from build123d import *

# Parameters (mm, degrees)
SKETCH1_W           = 32
SKETCH1_H           = 20
SKETCH1_R           = 1.6
BOSS_EXTRUDE1_DEPTH = 2
SKETCH3_W           = 40
SKETCH3_H           = 9
SKETCH3_R           = 1.45
BOSS_EXTRUDE2_DEPTH = 4
CUT_EXTRUDE1_DEPTH  = 2
FILLET1_R           = 10
CHAMFER1_SIZE       = 1
CUT_EXTRUDE2_REACH  = 28.019
SKETCH12_R          = 1.45
SKETCH12_R_2        = 0.95
FILLET2_R           = 1


with BuildPart() as part:
    # Sketch1 → Boss-Extrude1 (new body)
    with BuildSketch(Plane(origin=(0, 0, 0), x_dir=(1, 0, 0), z_dir=(0, 1, 0))):
        Rectangle(SKETCH1_W, SKETCH1_H)
        with Locations(Location((-5, 7.5, 0), (0, 0, 270))):
            Circle(SKETCH1_R, mode=Mode.SUBTRACT)
        with Locations(Location((5, 7.5, 0), (0, 0, 270))):
            Circle(SKETCH1_R, mode=Mode.SUBTRACT)
        with Locations(Location((-5, -7.5, 0), (0, 0, 270))):
            Circle(SKETCH1_R, mode=Mode.SUBTRACT)
        with Locations(Location((5, -7.5, 0), (0, 0, 270))):
            Circle(SKETCH1_R, mode=Mode.SUBTRACT)
    extrude(amount=BOSS_EXTRUDE1_DEPTH)

    # Sketch3 → Boss-Extrude2 (add)
    with BuildSketch(Plane.XY.offset(10)):
        with Locations((0, -2.5)):
            Rectangle(SKETCH3_W, SKETCH3_H)
        with Locations((0, -2.5)):
            Circle(SKETCH3_R, mode=Mode.SUBTRACT)
    extrude(amount=BOSS_EXTRUDE2_DEPTH)

    # Sketch4 → Cut-Extrude1 (cut)
    with BuildSketch(Plane(origin=(0, 0, 10), x_dir=(-1, 0, 0), z_dir=(0, 0, -1))):
        with BuildLine():
            Line((-16, 2), (-20, 2))
            Line((-20, 2), (-20, -7))
            Line((-20, -7), (20, -7))
            Line((20, -7), (20, 2))
            Line((20, 2), (16, 2))
            Line((16, 2), (16, 0))
            Line((16, 0), (4, 0))
            Line((4, 0), (4, -2.5))
            ThreePointArc((4, -2.5), (0, -6.5), (-4, -2.5))
            Line((-4, -2.5), (-4, 0))
            Line((-4, 0), (-16, 0))
            Line((-16, 0), (-16, 2))
        make_face()
    extrude(amount=-CUT_EXTRUDE1_DEPTH, mode=Mode.SUBTRACT)

    # Fillet1
    # the kernel refuses this fillet: 10 mm, written as the material it adds along each edge
    with BuildSketch(Plane(origin=(16, 0, 12), x_dir=(0, 0, -1), z_dir=(0, 1, 0)), Plane(origin=(-16, 2, 12), x_dir=(0, 0, -1), z_dir=(0, -1, 0))) as fillet1_piece_1:
        with BuildLine():
            CenterArc((8, -10), FILLET1_R, 90, 53.130102354)
            Line((0, -4), (-0.16, -3.88))
            ThreePointArc((-0.16, -3.88), (-0.2, -2), (-0.2, 0))
            Line((-0.2, 0), (0, 0.2))
            Line((0, 0.2), (8, 0.2))
            Line((8, 0.2), (8, 0))
        make_face()
    extrude(amount=2)

    # Chamfer1
    # the kernel refuses this chamfer: 1 mm, written as the material it takes off along each edge
    with BuildSketch(Plane(origin=(-5, 2, -7.5), x_dir=(0, 0, 1), z_dir=(-1, 0, 0))) as chamfer1_piece_1:
        Polygon((1.6 + CHAMFER1_SIZE, 0), (1.6, -CHAMFER1_SIZE), (1.6, 0), align=None)
    revolve(axis=Axis((-5, 2, -7.5), (0, 1, 0)), mode=Mode.SUBTRACT)
    with BuildSketch(Plane(origin=(5, 2, -7.5), x_dir=(0, 0, 1), z_dir=(-1, 0, 0))) as chamfer1_piece_2:
        Polygon((1.6 + CHAMFER1_SIZE, 0), (1.6, -CHAMFER1_SIZE), (1.6, 0), align=None)
    revolve(axis=Axis((5, 2, -7.5), (0, 1, 0)), mode=Mode.SUBTRACT)
    with BuildSketch(Plane(origin=(-5, 2, 7.5), x_dir=(0, 0, 1), z_dir=(-1, 0, 0))) as chamfer1_piece_3:
        Polygon((1.6 + CHAMFER1_SIZE, 0), (1.6, -CHAMFER1_SIZE), (1.6, 0), align=None)
    revolve(axis=Axis((-5, 2, 7.5), (0, 1, 0)), mode=Mode.SUBTRACT)
    with BuildSketch(Plane(origin=(5, 2, 7.5), x_dir=(0, 0, 1), z_dir=(-1, 0, 0))) as chamfer1_piece_4:
        Polygon((1.6 + CHAMFER1_SIZE, 0), (1.6, -CHAMFER1_SIZE), (1.6, 0), align=None)
    revolve(axis=Axis((5, 2, 7.5), (0, 1, 0)), mode=Mode.SUBTRACT)

    # Sketch12 → Cut-Extrude2 (cut, up to next)
    with BuildSketch(Plane(origin=(0, 2, 0), x_dir=(1, 0, 0), z_dir=(0, 1, 0)), mode=Mode.PRIVATE) as cut_extrude2_sk1:
        with Locations(Location((-13.5, 6, 0), (0, 0, 270))):
            Circle(SKETCH12_R)
    cut_extrude2_tool1 = extrude(cut_extrude2_sk1.sketch, amount=-CUT_EXTRUDE2_REACH, mode=Mode.PRIVATE) & part.part
    # Sketch12 → Cut-Extrude2 (cut, up to next)
    with BuildSketch(Plane(origin=(0, 2, 0), x_dir=(1, 0, 0), z_dir=(0, 1, 0)), mode=Mode.PRIVATE) as cut_extrude2_sk2:
        with Locations(Location((-13.5, -6, 0), (0, 0, 270))):
            Circle(SKETCH12_R)
    cut_extrude2_tool2 = extrude(cut_extrude2_sk2.sketch, amount=-CUT_EXTRUDE2_REACH, mode=Mode.PRIVATE) & part.part
    # Sketch12 → Cut-Extrude2 (cut, up to next)
    with BuildSketch(Plane(origin=(0, 2, 0), x_dir=(1, 0, 0), z_dir=(0, 1, 0)), mode=Mode.PRIVATE) as cut_extrude2_sk3:
        with Locations(Location((13.5, -6, 0), (0, 0, 270))):
            Circle(SKETCH12_R)
    cut_extrude2_tool3 = extrude(cut_extrude2_sk3.sketch, amount=-CUT_EXTRUDE2_REACH, mode=Mode.PRIVATE) & part.part
    # Sketch12 → Cut-Extrude2 (cut, up to next)
    with BuildSketch(Plane(origin=(0, 2, 0), x_dir=(1, 0, 0), z_dir=(0, 1, 0)), mode=Mode.PRIVATE) as cut_extrude2_sk4:
        with Locations(Location((13.5, 6, 0), (0, 0, 270))):
            Circle(SKETCH12_R)
    cut_extrude2_tool4 = extrude(cut_extrude2_sk4.sketch, amount=-CUT_EXTRUDE2_REACH, mode=Mode.PRIVATE) & part.part
    # Sketch12 → Cut-Extrude2 (cut, up to next)
    with BuildSketch(Plane(origin=(0, 2, 0), x_dir=(1, 0, 0), z_dir=(0, 1, 0)), mode=Mode.PRIVATE) as cut_extrude2_sk5:
        with Locations(Location((-9, 5.5, 0), (0, 0, 270))):
            Circle(SKETCH12_R_2)
    cut_extrude2_tool5 = extrude(cut_extrude2_sk5.sketch, amount=-CUT_EXTRUDE2_REACH, mode=Mode.PRIVATE) & part.part
    # Sketch12 → Cut-Extrude2 (cut, up to next)
    with BuildSketch(Plane(origin=(0, 2, 0), x_dir=(1, 0, 0), z_dir=(0, 1, 0)), mode=Mode.PRIVATE) as cut_extrude2_sk6:
        with Locations(Location((9, 5.5, 0), (0, 0, 270))):
            Circle(SKETCH12_R_2)
    cut_extrude2_tool6 = extrude(cut_extrude2_sk6.sketch, amount=-CUT_EXTRUDE2_REACH, mode=Mode.PRIVATE) & part.part
    # Sketch12 → Cut-Extrude2 (cut, up to next)
    with BuildSketch(Plane(origin=(0, 2, 0), x_dir=(1, 0, 0), z_dir=(0, 1, 0)), mode=Mode.PRIVATE) as cut_extrude2_sk7:
        with Locations(Location((9, -5.5, 0), (0, 0, 270))):
            Circle(SKETCH12_R_2)
    cut_extrude2_tool7 = extrude(cut_extrude2_sk7.sketch, amount=-CUT_EXTRUDE2_REACH, mode=Mode.PRIVATE) & part.part
    # Sketch12 → Cut-Extrude2 (cut, up to next)
    with BuildSketch(Plane(origin=(0, 2, 0), x_dir=(1, 0, 0), z_dir=(0, 1, 0)), mode=Mode.PRIVATE) as cut_extrude2_sk8:
        with Locations(Location((-9, -5.5, 0), (0, 0, 270))):
            Circle(SKETCH12_R_2)
    cut_extrude2_tool8 = extrude(cut_extrude2_sk8.sketch, amount=-CUT_EXTRUDE2_REACH, mode=Mode.PRIVATE) & part.part
    add(cut_extrude2_tool1.solids().sort_by_distance((-13.5, 2, -6))[0], mode=Mode.SUBTRACT)
    add(cut_extrude2_tool2.solids().sort_by_distance((-13.5, 2, 6))[0], mode=Mode.SUBTRACT)
    add(cut_extrude2_tool3.solids().sort_by_distance((13.5, 2, 6))[0], mode=Mode.SUBTRACT)
    add(cut_extrude2_tool4.solids().sort_by_distance((13.5, 2, -6))[0], mode=Mode.SUBTRACT)
    add(cut_extrude2_tool5.solids().sort_by_distance((-9, 2, -5.5))[0], mode=Mode.SUBTRACT)
    add(cut_extrude2_tool6.solids().sort_by_distance((9, 2, -5.5))[0], mode=Mode.SUBTRACT)
    add(cut_extrude2_tool7.solids().sort_by_distance((9, 2, 5.5))[0], mode=Mode.SUBTRACT)
    add(cut_extrude2_tool8.solids().sort_by_distance((-9, 2, 5.5))[0], mode=Mode.SUBTRACT)

    # Fillet2
    fillet2_edges = [part.edges().sort_by_distance(p)[0] for p in [
        (-16, 1, -10),
        (16, 1, -10),
    ]]
    fillet(fillet2_edges, radius=FILLET2_R)


solid = part.part
Can you work these out from the model? Positions are in its coordinate system, mm. A direction names the side the tool comes from. Coordinates: 2 decimals unless noted, no trailing zeros. Loops run counter-clockwise (first coordinate to the right, second up) from the corner with the lowest first, then second, coordinate; pieces in that order, holes last. Notation, with made-up numbers: M -28.5,88.5 L 7.5,88.5 A8 cw 7.5,97.5 Z; hole C 2,-10 d9. An arc over 180 degrees is marked long. Answer as CSV lines item,"result". Start each with the question number.
1. Thinking about a two-plate mould opening in Z: for faces 1 (the face through (0, 2, 2)), 2 (the face through (15.715, 1.014, -9.699)), 3 (the face through (-0.3, -4.4, 14)), 4 (the face through (12.62, 1.01, 4.85)), which applies, +Z half, -Z half, draft (parallel to the pull), parting line (faces both ways), or undercut?
2. Suppose I cut it at B-B, the plane x = 0. List the corners of the cut face in (y, z) for me.
3. For faces 5 (the face through (4, -1, 11)), 6 (the face through (-13.44, 1.01, 4.55)), 7 (the face through (16, 1, -3)), 8 (the face through (-16, 1, -3)), which set-ups out of +Z, -Z, +X, -X, +Y, -Y let a thin tool reach every point of the face, with its end or its side?
4. If I drill on probe 1 along X at (y, z) = (0.55, -7.5); probe 2 along X at (y, z) = (0.55, 5.5); probe 3 along X at (y, z) = (0.8, -5.5), over which ranges is the centre line in solid material (lowest first)? Write a range as [from, to].
5. Suppose I cut it at D-D, the plane x = -5. List the corners of the cut face in (y, z) for me.
6. For pin 1 Ø3.5 at (x, z) = (5, 7.5) entering from +Y; pin 2 Ø3 at (x, z) = (-9, 5.5) entering from -Y; pin 3 Ø2 at (y, z) = (0.5, -5) entering from -X, each with a flat end and sliding along its axis, tell me the tip position at first contact or that it passes through.
7. Suppose I cut it at A-A, the plane x = -9. List the corners of the cut face in (y, z) for me.
8. Suppose I cut it at C-C, the plane y = -1.5. List the corners of the cut face in (x, z) for me, plus the area to 3 significant figures.
Output:
1,face 1,"draft"
1,face 2,"-Z half"
1,face 3,"+Z half"
1,face 4,"undercut"
2,outline,"M -7,12 L -6.5,12 L -6.5,10 L -3.95,10 L -3.95,14 L -7,14 Z; M -1.05,10 L 0,10 L 0,-10 L 2,-10 L 2,14 L -1.05,14 Z"
3,face 5,"-Z, +X, -Y"
3,face 6,"+Y, -Y"
3,face 7,"-Z, +X, +Y, -Y"
3,face 8,"-Z, -X, +Y, -Y"
4,probe 1,"x = [-16, -6.6], [-3.4, 3.4], [6.6, 16]"
4,probe 2,"x = [-16.11, -14.86], [-12.14, -9.95], [-8.05, 8.05], [9.95, 12.14], [14.86, 16.11]"
4,probe 3,"x = [-16, -14.86], [-12.14, -9.95], [-8.05, 8.05], [9.95, 12.14], [14.86, 16]"
5,outline,"M -7,12 L 0,12 L 0,9.1 L 1,9.1 L 2,10.1 L 2,14 L -7,14 Z; M 0,-10 L 1.9,-10 L 1,-9.1 L 0,-9.1 Z; M 0,-5.9 L 1,-5.9 L 2,-4.9 L 2,4.9 L 1,5.9 L 0,5.9 Z"
6,pin 1,"stops at y = 1.15"
6,pin 2,"stops at y = 0"
6,pin 3,"stops at x = -16"
7,outline,"M -7,12 L 0,12 L 0,6.45 L 2,6.45 L 2,14 L -7,14 Z; M 0,-10 L 2,-10 L 2,-6.45 L 0,-6.45 Z; M 0,-4.55 L 2,-4.55 L 2,4.55 L 0,4.55 Z"
8,outline,"M -20,12 L -4,12 L -4,10 L -1.05,10 L -1.05,14 L -20,14 Z; M 1.05,10 L 4,10 L 4,12 L 20,12 L 20,14 L 1.05,14 Z"
8,area,"87.6 mm^2"
